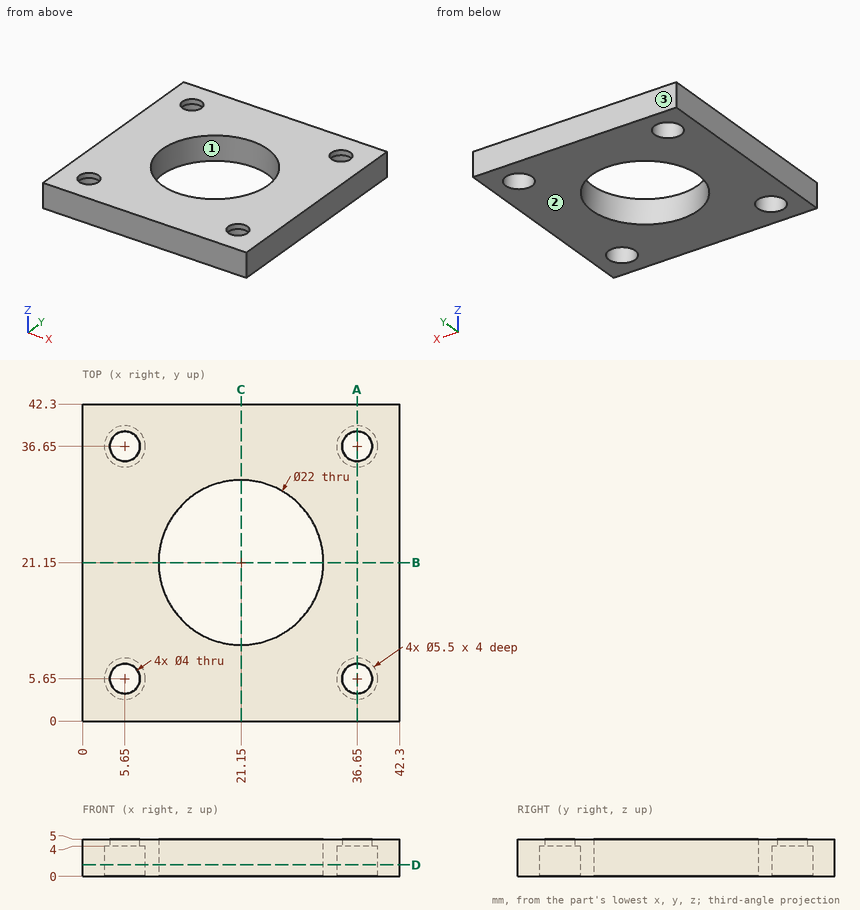
Can you work these out from the drawing? Everything is in mm from the part's minimum corner. Give positions to 0.01 mm unless a question says otherwise; leave off trailing zeros. Loops run counter-clockwise (first coordinate to the right, second up) from the corner with the lowest first, then second, coordinate; pieces in that order, holes last. Notation, with made-up numbers: M 6.25,-36.75 L 54.25,-36.75 A14 ccw 54.25,-32.75 Z; hole C 1.5,-39.75 d1. An arc over 180 degrees is marked long. Put each result on its own line as item: value. Start each with the question number.
(1) I need wall thicknesses on line 1 along Y through (x, z) = (36.65, 1.05); line 2 along Y through (x, z) = (36.65, 4.8); line 3 along Y through (x, z) = (21, 3.9). Which ranges of each line are inside material? Lowest first, please. Write a range as [from, to].
(2) If we mould it in two halves opening along Y, with no side actions, what happens to the marked faces 1, 2 and 3? For each: +Y half, -Y half, draft (parallel to the pull), parting line (faces both ways), or undercut.
(3) I want a section at B-B on y = 21.15. Please give me the cut outline in (x, z), then the cut area to 4 significant figures.
(4) I want a section at D-D on z = 1.55. Please give me the cut outline in (x, y), then the cut area to 3 significant figures.
(5) Will this pin go through, and if not, where does the flat tip stop? pin 1 Ø17.5 at (x, y) = (21.15, 21.15) entering from +Z.
(6) I want a section at A-A on x = 36.65. Please give me the cut outline in (y, z).
Answer block:
1. line 1: [0, 2.9], [8.4, 33.9], [39.4, 42.3]
1. line 2: [0, 3.65], [7.65, 34.65], [38.65, 42.3]
1. line 3: [0, 10.15], [32.15, 42.3]
2. face 1: undercut
2. face 2: draft
2. face 3: +Y half
3. outline: M 0,0 L 10.15,0 L 10.15,5 L 0,5 Z; M 32.15,0 L 42.3,0 L 42.3,5 L 32.15,5 Z
3. area: 101.5 mm^2
4. outline: M 0,0 L 42.3,0 L 42.3,42.3 L 0,42.3 Z; hole C 5.65,5.65 d5.5; hole C 5.65,36.65 d5.5; hole C 21.15,21.15 d22; hole C 36.65,5.65 d5.5; hole C 36.65,36.65 d5.5
4. area: 1,310 mm^2
5. pin 1: through
6. outline: M 0,0 L 2.9,0 L 2.9,4 L 3.65,4 L 3.65,5 L 0,5 Z; M 7.65,4 L 8.4,4 L 8.4,0 L 33.9,0 L 33.9,4 L 34.65,4 L 34.65,5 L 7.65,5 Z; M 38.65,4 L 39.4,4 L 39.4,0 L 42.3,0 L 42.3,5 L 38.65,5 Z
